Input: part model. Units: mm. Frame: model coordinates. A direction names the side the tool comes from. Coordinates: 2 decimals unless noted, no trailing zeros. Order: outer loops, then holes, each group sorted by start corner. A loop starts at its lowest first (then second) coordinate and runs counter-clockwise, first axis right, second up. Notation, with made-up numbers: (70, 43.25) -> (84, 43.25) arc R19 cw to (84, 47.25) -> close; hole circle Ø5 at (-36.5, -36). An arc over 180 degrees is marked (long way). Write each question's results on one line, items separated by ' | '.
```python
from build123d import *
from build123d import SkipClean  # not in build123d's __all__

# Parameters (mm, degrees)
F1_DEPTH = 10
F0_R     = 24.5
F2_DEPTH = 30
F3_DEPTH = 20
F4_DEPTH = 20
F5_DEPTH = 30
F6_DEPTH = 5


with BuildPart() as f1:
    # F0 (on Top) → F1 (new body)
    with BuildSketch(Plane.XY):
        with BuildLine():
            ThreePointArc((-9.06851449, 27.018735073), (0, 28.5), (9.06851449, 27.018735073))
            Line((9.06851449, 27.018735073), (9.8690700263, 29.3870967742))
            ThreePointArc((9.8690700263, 29.3870967742), (0, 31), (-9.8690700263, 29.3870967742))
            Line((-9.8690700263, 29.3870967742), (-9.06851449, 27.018735073))
        make_face()
        with BuildLine():
            ThreePointArc((-9.06851449, -27.018735073), (-28.5, 0), (-9.06851449, 27.018735073))
            Line((-9.06851449, 27.018735073), (-9.8690700263, 29.3870967742))
            ThreePointArc((-9.8690700263, 29.3870967742), (-31, 0), (-9.8690700263, -29.3870967742))
            Line((-9.8690700263, -29.3870967742), (-9.06851449, -27.018735073))
        make_face()
        with BuildLine():
            Line((9.8690700263, -29.3870967742), (9.06851449, -27.018735073))
            ThreePointArc((9.06851449, -27.018735073), (0, -28.5), (-9.06851449, -27.018735073))
            Line((-9.06851449, -27.018735073), (-9.8690700263, -29.3870967742))
            ThreePointArc((-9.8690700263, -29.3870967742), (0, -31), (9.8690700263, -29.3870967742))
        make_face()
        with BuildLine():
            ThreePointArc((9.06851449, 27.018735073), (23.1376604583, 16.6402724893), (28.5, 0))
            ThreePointArc((28.5, 0), (23.1376604583, -16.6402724893), (9.06851449, -27.018735073))
            Line((9.06851449, -27.018735073), (9.8690700263, -29.3870967742))
            ThreePointArc((9.8690700263, -29.3870967742), (25.1688415587, -18.0977737469), (31, 0))
            ThreePointArc((31, 0), (25.1688415587, 18.0977737469), (9.8690700263, 29.3870967742))
            Line((9.8690700263, 29.3870967742), (9.06851449, 27.018735073))
        make_face()
    extrude(amount=F1_DEPTH)

    # F0 (on Top) → F2 (cut)
    with BuildSketch(Plane.XY):
        with BuildLine():
            ThreePointArc((9.06851449, -27.018735073), (23.1376604583, -16.6402724893), (28.5, 0))
            ThreePointArc((28.5, 0), (23.1376604583, 16.6402724893), (9.06851449, 27.018735073))
            ThreePointArc((9.06851449, 27.018735073), (0, 28.5), (-9.06851449, 27.018735073))
            ThreePointArc((-9.06851449, 27.018735073), (-28.5, 0), (-9.06851449, -27.018735073))
            ThreePointArc((-9.06851449, -27.018735073), (0, -28.5), (9.06851449, -27.018735073))
        make_face()
        Circle(F0_R, mode=Mode.SUBTRACT)
    extrude(amount=F2_DEPTH, mode=Mode.SUBTRACT)

    # F0 (on Top) → F3 (join)
    with BuildSketch(Plane.XY):
        with BuildLine():
            ThreePointArc((-9.06851449, 27.018735073), (0, 28.5), (9.06851449, 27.018735073))
            Line((9.06851449, 27.018735073), (9.8690700263, 29.3870967742))
            ThreePointArc((9.8690700263, 29.3870967742), (0, 31), (-9.8690700263, 29.3870967742))
            Line((-9.8690700263, 29.3870967742), (-9.06851449, 27.018735073))
        make_face()
    with SkipClean():  # cleaning this boolean's faces spoils the solid; the shape is the same uncleaned
        extrude(amount=F3_DEPTH)

    # F0 (on Top) → F4 (join)
    with BuildSketch(Plane.XY):
        with BuildLine():
            Line((9.8690700263, -29.3870967742), (9.06851449, -27.018735073))
            ThreePointArc((9.06851449, -27.018735073), (0, -28.5), (-9.06851449, -27.018735073))
            Line((-9.06851449, -27.018735073), (-9.8690700263, -29.3870967742))
            ThreePointArc((-9.8690700263, -29.3870967742), (0, -31), (9.8690700263, -29.3870967742))
        make_face()
    with SkipClean():  # cleaning this boolean's faces spoils the solid; the shape is the same uncleaned
        extrude(amount=F4_DEPTH)

    # F0 (on Top) → F5 (join)
    with BuildSketch(Plane.XY):
        with BuildLine():
            ThreePointArc((9.06851449, -27.018735073), (23.1376604583, -16.6402724893), (28.5, 0))
            ThreePointArc((28.5, 0), (23.1376604583, 16.6402724893), (9.06851449, 27.018735073))
            ThreePointArc((9.06851449, 27.018735073), (0, 28.5), (-9.06851449, 27.018735073))
            ThreePointArc((-9.06851449, 27.018735073), (-28.5, 0), (-9.06851449, -27.018735073))
            ThreePointArc((-9.06851449, -27.018735073), (0, -28.5), (9.06851449, -27.018735073))
        make_face()
        Circle(F0_R, mode=Mode.SUBTRACT)
    extrude(amount=F5_DEPTH)

    # F0 (on Top) → F6 (join)
    with BuildSketch(Plane.XY):
        Circle(F0_R)
    extrude(amount=F6_DEPTH)


solid = f1.part
```
(1) Cut plane C-C, the plane y = 5. Return loops of the section in (x, z), plus the area to 3 significant figures.
Return value:
outline: (-30.59, 0) -> (30.59, 0) -> (30.59, 10) -> (28.06, 10) -> (28.06, 30) -> (23.98, 30) -> (23.98, 5) -> (-23.98, 5) -> (-23.98, 30) -> (-28.06, 30) -> (-28.06, 10) -> (-30.59, 10) -> close | area: 535 mm2
(2) Reachability of faces 4 (the face through (-9.463, -28.186, 14.93)), 5 (the face through (0, 0, 5)), 6 (the face through (9.474, -28.219, 14.93)) from +Z, -Z, +X, -X, +Y, -Y: full face, straight path, thin tool, end or side. Return the list, or none.
Return value:
face 4: +Z, -X | face 5: +Z | face 6: +Z, +X
(3) Cut plane B-B, the plane z = 18.75. Return loops of the section in (x, y).
Return value:
outline: (-9.87, -29.39) arc R31 ccw to (9.87, -29.39) -> (9.07, -27.02) arc R28.5 ccw to (9.07, 27.02) -> (9.87, 29.39) arc R31 ccw to (-9.87, 29.39) -> (-9.07, 27.02) arc R28.5 ccw to (-9.07, -27.02) -> close; hole circle Ø49 at (0, 0)
(4) Mould query, pull axis Y, two halves, no side actions, for faces 1 (the face through (13.17, 20.66, 17.32)), 2 (the face through (0, 29, 20)), 3 (the face through (-0.586, -30.994, 5.416)). Classes: +Y half, -Y half, draft (parallel to the pull), parting line (faces both ways), or undercut.
Return value:
face 1: undercut | face 2: draft | face 3: parting line
(5) Cut plane D-D, the plane z = 8.5. Return loops of the section in (x, y), plus the area to 3 significant figures.
Return value:
outline: circle Ø62 at (0, 0); hole circle Ø49 at (0, 0) | area: 1,130 mm2
(6) Cut plane A-A, the plane x = 0. Return loops of the section in (y, z).
Return value:
outline: (-31, 0) -> (31, 0) -> (31, 20) -> (28.5, 20) -> (28.5, 30) -> (24.5, 30) -> (24.5, 5) -> (-24.5, 5) -> (-24.5, 30) -> (-28.5, 30) -> (-28.5, 20) -> (-31, 20) -> close
(7) Line query: line 1 along Y through (x, z) = (0, 12.25); line 2 along Y through (x, z) = (0, 21.5); line 3 along Z through (x, y) = (18, -11.5). Output: solid intervals per line, ascending. Write a range as from..to.
Return value:
line 1: -31..-24.5, 24.5..31 | line 2: -28.5..-24.5, 24.5..28.5 | line 3: 0..5
(8) Pin query (flat end, axial travel): P1, Ø5, axis at y = 0.5, z = 21, coming from the +X side; P2, Ø8, axis at x = 18, y = -18, coming from the -Z side; P3, Ø1.5, axis at x = 11.5, z = 24, coming from the +Y side; P4, Ø12, axis at y = 24, z = 26.5, coming from the -X side. Return the tip coordinate at first contact, or that it passes through.
Return value:
P1: x = 28.5 | P2: z = 0 | P3: y = 26.39 | P4: x = -22.1
